Verification items for the finished model (mm, model axes). Face numbers are marked on the shaded views. Coordinates: 2 decimals unless noted, no trailing zeros. Write each loop counter-clockwise with the first axis right and the second up, starting at its lowest first coordinate (ties: lowest second). Pieces come first, ordered by that corner, then holes. Notation, with made-up numbers: (31.25, 10) - (79.25, 10) arc R19 ccw to (79.25, 17) - close; hole circle Ø6 at (31, -32.75). An arc over 180 degrees is marked (long way). Answer as CSV lines item,"result". Start each with the question number.
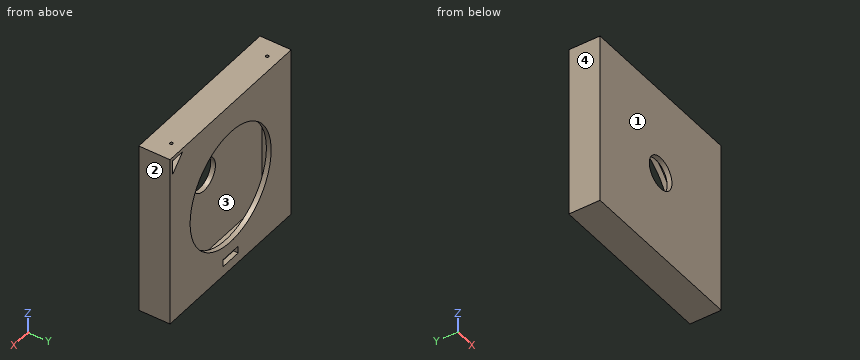
```python
from build123d import *

# Parameters (mm, degrees)
SKETCH1_W               = 304.8
SKETCH1_H               = 304.8
BOSS_EXTRUDE1_DEPTH     = 54.77002
SKETCH2_R               = 101.854
SKETCH2_W               = 38.1
SKETCH2_H               = 12.7
CUT_EXTRUDE3_DEPTH      = 38.1
SKETCH3_R               = 2.54
CUT_EXTRUDE4_DEPTH      = 31.75
CUT_EXTRUDE5_DEPTH      = 19.05
CUT_EXTRUDE5_DEPTH_BACK = 19.05
SKETCH4_W               = 292.1
SKETCH4_H               = 292.1
SKETCH5_R               = 28.448
CUT_EXTRUDE6_DEPTH      = 273.928796473


with BuildPart() as part:
    # Sketch1 → Boss-Extrude1 (new body)
    with BuildSketch(Plane(origin=(0, 0, 0), x_dir=(1, 0, 0), z_dir=(0, 1, 0))):
        with Locations((13.737464789, -57.096338028)):
            Rectangle(SKETCH1_W, SKETCH1_H)
    extrude(amount=BOSS_EXTRUDE1_DEPTH)

    # Sketch2 → Cut-Extrude3 (cut)
    with BuildSketch(Plane(origin=(0, 54.77002, 0), x_dir=(1, 0, 0), z_dir=(0, 1, 0))):
        with Locations(Location((13.737464789, -57.096338028, 0), (0, 0, 270))):
            Circle(SKETCH2_R)
        Polygon((134.387464789, -203.146338028), (159.787464789, -203.146338028), (159.787464789, -177.746338028), align=None)
        with Locations((13.737464789, 71.941420767)):
            Rectangle(SKETCH2_W, SKETCH2_H)
    extrude(amount=-CUT_EXTRUDE3_DEPTH, mode=Mode.SUBTRACT)

    # Sketch3 → Cut-Extrude4 (cut)
    with BuildSketch(Plane.XY.offset(209.496338028)):
        with Locations((134.387464789, 34.95802)):
            Circle(SKETCH3_R)
        with Locations((-106.912535211, 34.95802)):
            Circle(SKETCH3_R)
    extrude(amount=-CUT_EXTRUDE4_DEPTH, mode=Mode.SUBTRACT)

    # Sketch4 → Cut-Extrude5 (cut, two sides: drawn at the far end of the back side and taken through both)
    with BuildSketch(Plane(origin=(0, 27.38501, 0), x_dir=(1, 0, 0), z_dir=(0, 1, 0)).offset(-CUT_EXTRUDE5_DEPTH_BACK)):
        with Locations((13.737464789, -57.096338028)):
            Rectangle(SKETCH4_W, SKETCH4_H)
    extrude(amount=CUT_EXTRUDE5_DEPTH + CUT_EXTRUDE5_DEPTH_BACK, mode=Mode.SUBTRACT)

    # Sketch5 → Cut-Extrude6 (cut, through all)
    with BuildSketch(Plane.XZ):
        with Locations(Location((13.737464789, 57.096338028, 0), (0, 0, 270))):
            Circle(SKETCH5_R)
    extrude(amount=-CUT_EXTRUDE6_DEPTH, mode=Mode.SUBTRACT)


solid = part.part
```
1. Cross-section at A-A (x = -99). Record the cut outline in (y, z) (3 decimals), and give its area (3 significant figures).
2. Cross-section at D-D (z = 70.5). Record the cut outline in (x, y) (3 decimals), and give its area (3 significant figures).
3. Scan lines: line 1 along Y through (x, z) = (-126, 35); line 2 along X through (y, z) = (10, 9.5); line 3 along Z through (x, y) = (1, 23). Record each from-to range of solid material in increasing order. Write a range as from..to.
4. Depth check by flat-ended pin: P1, Ø4.5, axis at x = 134.39, y = 34.96, coming from the +Z side. Enter the tip coordinate at first touch or a pass-through.
5. Cross-section at C-C (x = -1.5). Record the cut outline in (y, z) (3 decimals).
6. Cross-section at B-B (y = 41.5). Record the cut outline in (x, z).
7. Draft check along X on the marked faces 1, 2, 3 and 4. Enter one of: pulls with the +X half, pulls with the -X half, needs draft (parallel to the pull), parting line crosses it, or undercut.
Completed:
1,outline,"(0, -95.304) - (54.77, -95.304) - (54.77, 209.496) - (0, 209.496) - close; hole (8.335, -88.954) - (46.435, -88.954) - (46.435, 203.146) - (8.335, 203.146) - close"
1,area,"5,560 mm2"
2,outline,"(-138.663, 0) - (-11.355, 0) - (-11.355, 8.335) - (-132.313, 8.335) - (-132.313, 46.435) - (-87.231, 46.435) - (-87.231, 54.77) - (-138.663, 54.77) - close; (38.83, 0) - (166.137, 0) - (166.137, 54.77) - (114.706, 54.77) - (114.706, 46.435) - (159.787, 46.435) - (159.787, 8.335) - (38.83, 8.335) - close"
2,area,"3,460 mm2"
3,line 1,"y = 0..8.34, 46.44..54.77"
3,line 2,"x = -138.66..-132.31, 159.79..166.14"
3,line 3,"z = -95.3..-88.95, 203.15..209.5"
4,P1,"stops at z = -88.95"
5,outline,"(0, -95.304) - (54.77, -95.304) - (54.77, -78.291) - (46.435, -78.291) - (46.435, -88.954) - (8.335, -88.954) - (8.335, 33.073) - (0, 33.073) - close; (0, 81.119) - (8.335, 81.119) - (8.335, 203.146) - (46.435, 203.146) - (46.435, 157.804) - (54.77, 157.804) - (54.77, 209.496) - (0, 209.496) - close; (46.435, -65.591) - (54.77, -65.591) - (54.77, -43.611) - (46.435, -43.611) - close"
6,outline,"(-138.66, -95.3) - (166.14, -95.3) - (166.14, 209.5) - (-138.66, 209.5) - close; hole (-132.31, -88.95) - (159.79, -88.95) - (159.79, 203.15) - (-132.31, 203.15) - close"
7,face 1,"needs draft"
7,face 2,"pulls with the +X half"
7,face 3,"undercut"
7,face 4,"pulls with the -X half"
